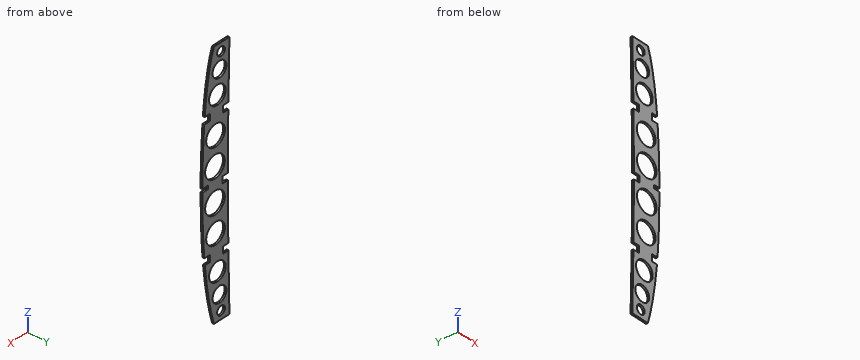
```python
from build123d import *

# Parameters (mm, degrees)
F0_R     = 20.913693
F0_R_2   = 17.465472
F0_R_3   = 9.869676
F0_R_4   = 24.682403
F0_R_5   = 23.589378
F1_DEPTH = 4


with BuildPart() as f1:
    # F0 (on Front) → F1 (new body)
    with BuildSketch(Plane.XZ):
        with BuildLine():
            Line((-105.642843, 354.427334), (-144.642843, 354.427334))
            add(Edge.make_bspline(
                [(-144.642843, 354.427334), (-143.713265, 310.427334), (-142.783688, 266.427334), (-142.054926, 222.427334)],
                knots=[0, 0, 0, 0, 132.013092, 132.013092, 132.013092, 132.013092], degree=3))
            Line((-142.054926, 222.427334), (-128.054926, 222.427334))
            Line((-128.054926, 222.427334), (-128.054926, 214.927334))
            Line((-128.054926, 214.927334), (-95.232242, 214.927334))
            Line((-95.232242, 214.927334), (-95.232242, 222.427334))
            Line((-95.232242, 222.427334), (-82.397624, 222.427334))
            add(Edge.make_bspline(
                [(-105.642843, 354.427334), (-94.373968, 324.244912), (-86.922567, 276.685565), (-82.397624, 222.427334)],
                knots=[0, 0, 0, 0, 151.629613, 151.629613, 151.629613, 151.629613], degree=3))
        make_face()
        with Locations((-114.42259, 251.343668)):
            Circle(F0_R, mode=Mode.SUBTRACT)
        with Locations((-119.738169, 301.082313)):
            Circle(F0_R_2, mode=Mode.SUBTRACT)
        with Locations((-123.535015, 336.013287)):
            Circle(F0_R_3, mode=Mode.SUBTRACT)
        with BuildLine():
            Line((-128.054926, 207.427334), (-141.814558, 207.427334))
            add(Edge.make_bspline(
                [(-141.814558, 207.427334), (-141.146919, 164.260708), (-140.694523, 121.094083), (-140.646991, 77.927458)],
                knots=[147.01458, 147.01458, 147.01458, 147.01458, 276.5273, 276.5273, 276.5273, 276.5273], degree=3))
            add(Edge.make_bspline(
                [(-140.646991, 77.927458), (-140.646991, 77.927416), (-140.646991, 77.927375), (-140.646991, 77.927334)],
                knots=[276.5273, 276.5273, 276.5273, 276.5273, 276.527424, 276.527424, 276.527424, 276.527424], degree=3))
            Line((-140.646991, 77.927334), (-126.646991, 77.927334))
            Line((-126.646991, 77.927334), (-126.646991, 70.427334))
            Line((-126.646991, 70.427334), (-90.667988, 70.427334))
            Line((-90.667988, 70.427334), (-90.661724, 70.427334))
            Line((-90.661724, 70.427334), (-90.661724, 77.927334))
            Line((-90.661724, 77.927334), (-76.661724, 77.927334))
            add(Edge.make_bspline(
                [(-81.232242, 207.427334), (-78.239795, 165.975298), (-76.840765, 121.316902), (-76.661724, 77.927334)],
                knots=[165.454488, 165.454488, 165.454488, 165.454488, 278.926983, 278.926983, 278.926983, 278.926983], degree=3))
            Line((-81.232242, 207.427334), (-95.232242, 207.427334))
            Line((-95.232242, 207.427334), (-95.232242, 214.927334))
            Line((-95.232242, 214.927334), (-128.054926, 214.927334))
            Line((-128.054926, 214.927334), (-128.054926, 207.427334))
        make_face()
        with Locations((-108.347639, 107.443303)):
            Circle(F0_R_4, mode=Mode.SUBTRACT)
        with Locations((-109.866373, 170.85059)):
            Circle(F0_R_5, mode=Mode.SUBTRACT)
        with BuildLine():
            add(Edge.make_bspline(
                [(-142.054926, -81.572666), (-142.783688, -125.572666), (-143.713265, -169.572666), (-144.642843, -213.572666)],
                knots=[436.043243, 436.043243, 436.043243, 436.043243, 568.056335, 568.056335, 568.056335, 568.056335], degree=3))
            Line((-144.642843, -213.572666), (-105.642843, -213.572666))
            add(Edge.make_bspline(
                [(-82.791095, -81.572666), (-87.337348, -130.326688), (-94.669187, -174.905471), (-105.642843, -213.572666)],
                knots=[426.00823, 426.00823, 426.00823, 426.00823, 570.953588, 570.953588, 570.953588, 570.953588], degree=3))
            Line((-82.791095, -81.572666), (-95.232242, -81.572666))
            Line((-95.232242, -81.572666), (-95.232242, -74.072666))
            Line((-95.232242, -74.072666), (-95.232242, -66.572666))
            Line((-95.232242, -66.572666), (-81.489773, -66.572666))
            add(Edge.make_bspline(
                [(-76.642843, 70.427334), (-76.599115, 22.505564), (-78.028195, -23.539434), (-81.489773, -66.572666)],
                knots=[285.476794, 285.476794, 285.476794, 285.476794, 411.269799, 411.269799, 411.269799, 411.269799], degree=3))
            Line((-76.642843, 70.427334), (-90.661724, 70.427334))
            Line((-90.661724, 70.427334), (-90.667988, 70.427334))
            Line((-90.667988, 70.427334), (-126.646991, 70.427334))
            Line((-126.646991, 70.427334), (-126.646991, 62.927334))
            Line((-126.646991, 62.927334), (-140.646991, 62.927334))
            add(Edge.make_bspline(
                [(-140.646991, 62.927334), (-140.694522, 19.760667), (-141.146918, -23.405999), (-141.814558, -66.572666)],
                knots=[291.528911, 291.528911, 291.528911, 291.528911, 421.041756, 421.041756, 421.041756, 421.041756], degree=3))
            Line((-141.814558, -66.572666), (-128.054926, -66.572666))
            Line((-128.054926, -66.572666), (-128.054926, -74.072666))
            Line((-128.054926, -74.072666), (-128.054926, -81.572666))
            Line((-128.054926, -81.572666), (-142.054926, -81.572666))
        make_face()
        with Locations((-123.535015, -195.158619)):
            Circle(F0_R_3, mode=Mode.SUBTRACT)
        with Locations((-119.738169, -160.227645)):
            Circle(F0_R_2, mode=Mode.SUBTRACT)
        with Locations((-114.42259, -110.489)):
            Circle(F0_R, mode=Mode.SUBTRACT)
        with Locations((-109.866373, -29.995922)):
            Circle(F0_R_5, mode=Mode.SUBTRACT)
        with Locations((-108.347639, 33.411365)):
            Circle(F0_R_4, mode=Mode.SUBTRACT)
    extrude(amount=F1_DEPTH)


solid = f1.part
```
Geometry: final body of the model. Coordinates: model frame, mm. Round coordinates to 2 decimals unless told otherwise and drop trailing zeros. One line per item, written item: value.
(1) Pin query (flat end, axial travel): P1, Ø2, axis at y = -3, z = -72, coming from the -X side; P2, Ø1, axis at y = -1, z = 208, coming from the +X side; P3, Ø4, axis at x = -112, z = 233, coming from the -Y side; P4, Ø1.2, axis at y = -2, z = 72, coming from the -X side. Return the tip coordinate at first contact, or that it passes through.
Result sheet:
P1: x = -128.05
P2: x = -95.23
P3: through
P4: x = -126.65
(2) Line query: probe 1 along Z at (x, y) = (-137.5, -0.35); probe 2 along X at (y, z) = (-3.1, 23.5); probe 3 along X at (y, z) = (-3.25, -93.5). Output: solid intervals per line, ascending. Write a range as [from, to].
Result sheet:
probe 1: [-213.57, -81.57], [-66.57, 62.93], [77.93, 207.43], [222.43, 354.43]
probe 2: [-140.8, -130.95], [-85.74, -77.1]
probe 3: [-142.26, -126.62], [-102.23, -83.97]
(3) Cut plane A-A (x = -119). Give the number of separate pieces and of enclosed holes in the cut face, and give its area (3 significant figures).
Result sheet:
separate pieces: 11
enclosed holes: 0
area: 822 mm2
